Source: CAD feature listing. Evaluate the final solid. Frame: model axes, mm. A direction names the side the tool comes from. Round coordinates to 2 decimals unless told otherwise and drop trailing zeros. Order: outer loops, then holes, each group sorted by start corner. A loop starts at its lowest first (then second) coordinate and runs counter-clockwise, first axis right, second up. Notation, with made-up numbers: (-23, -10) -> (-2, -10) arc R23 ccw to (-2, 20) -> close; hole circle Ø8 at (73, 82). An arc over 180 degrees is marked (long way). One line per item, written item: value. Start each with the question number.
1) Section A-A (x = -15). Return the cut outline in (y, z).
2) Ray query, L1, parallel to Y at x = -4.5, z = 1.7; L2, parallel to X at y = 20, z = 4.25; L3, parallel to Z at x = -1, y = 18.5. Return the intervals inside material, ascending.
3) Pin query (flat end, axial travel): P1, Ø6, axis at y = 41, z = 3.5, coming from the +X side; P2, Ø2.5, axis at x = -75.5, z = 1.5, coming from the +Y side; P3, Ø4, axis at y = 96.5, z = 8.5, coming from the -X side. Return the tip coordinate at first contact, or that it passes through.
4) Section B-B (z = 10.5). Return the cut outline in (x, y), and give its area (3 significant figures).
5) Section C-C (y = 67). Return the cut outline in (x, z).
6) Reachability of faces 4 (the face through (0, 48, 2)), 5 (the face through (-5, 93.4, 8)), 6 (the face through (-24.5, 96, 8)) from +Z, -Z, +X, -X, +Y, -Y: full face, straight path, thin tool, end or side. Return the list, or none.
7) Section D-D (x = -125). Return the cut outline in (y, z), and give its area (3 significant figures).
8) Mould query, pull axis Y, two halves, no side actions, for faces 1 (the face through (15.5, 96, 8)), 2 (the face through (-180.285, 3.665, 8.944)), 3 (the face through (-9, 52, 2)). Classes: pulls with the +Y half, pulls with the -Y half, needs draft (parallel to the pull), parting line crosses it, or undercut.
```python
from build123d import *

# Parameters (mm, degrees)
F1_DEPTH = 5
F2_W     = 40
F2_H     = 5
F3_DEPTH = 12
F4_R     = 2.18125
F5_DEPTH = 8
F6_R     = 2.5
F7_DEPTH = 25


with BuildPart() as f1:
    # F0 (on Top) → F1 (new body)
    with BuildSketch(Plane.XY):
        with BuildLine():
            Line((15.5, 98.4), (-24.5, 98.4))
            Line((-24.5, 98.4), (-24.5, 93.4))
            Line((-24.5, 93.4), (-9, 93.4))
            Line((-9, 93.4), (-9, 9))
            Line((-9, 9), (-182.3, 9))
            ThreePointArc((-182.3, 9), (-186.8, 4.5), (-182.3, 0))
            Line((-182.3, 0), (-4.5, 0))
            ThreePointArc((-4.5, 0), (-1.318019, 1.318019), (0, 4.5))
            Line((0, 4.5), (0, 93.4))
            Line((0, 93.4), (15.5, 93.4))
            Line((15.5, 93.4), (15.5, 98.4))
        make_face()
    extrude(amount=F1_DEPTH)

    # F2 (on face) → F3 (join)
    with BuildSketch(Plane.XY.offset(5)):
        with Locations((-4.5, 95.9)):
            Rectangle(F2_W, F2_H)
    extrude(amount=F3_DEPTH)

    # F4 (on face) → F5 (join)
    with BuildSketch(Plane.XY.offset(5)):
        with Locations((-182.3, 4.5)):
            Circle(F4_R)
    extrude(amount=F5_DEPTH)

    # F6 (on face) → F7 (cut)
    with BuildSketch(Plane.XY.offset(5)):
        with Locations((-4.5, 4.5)):
            Circle(F6_R)
    extrude(amount=-F7_DEPTH, mode=Mode.SUBTRACT)


solid = f1.part
```
Findings:
1. outline: (0, 0) -> (9, 0) -> (9, 5) -> (0, 5) -> close; (93.4, 0) -> (98.4, 0) -> (98.4, 17) -> (93.4, 17) -> close
2. L1: 0 to 2, 7 to 98.4
2. L2: -9 to 0
2. L3: 0 to 5
3. P1: x = 0
3. P2: y = 9
3. P3: x = -24.5
4. outline: circle Ø4.36 at (-182.3, 4.5); (-24.5, 93.4) -> (15.5, 93.4) -> (15.5, 98.4) -> (-24.5, 98.4) -> close
4. area: 215 mm2
5. outline: (-9, 0) -> (0, 0) -> (0, 5) -> (-9, 5) -> close
6. face 4: +Z, -Z, +X, -Y
6. face 5: +Z
6. face 6: +Z, -Z, -X, +Y
7. outline: (0, 0) -> (9, 0) -> (9, 5) -> (0, 5) -> close
7. area: 45.0 mm2
8. face 1: needs draft
8. face 2: parting line crosses it
8. face 3: undercut
